Read the model definition and answer for the solid it produces. Units are mm, in the model's axes. Round coordinates to 2 decimals unless told otherwise and drop trailing zeros. Loops run counter-clockwise (first coordinate to the right, second up) from the corner with the lowest first, then second, coordinate; pieces in that order, holes last. Notation, with made-up numbers: (-37.75, 32) -> (-33.75, 32) arc R13 cw to (-33.75, 38) -> close; hole circle Ø9 at (40.25, -36.75). An arc over 180 degrees is marked (long way). Put each result on its own line as item: value.
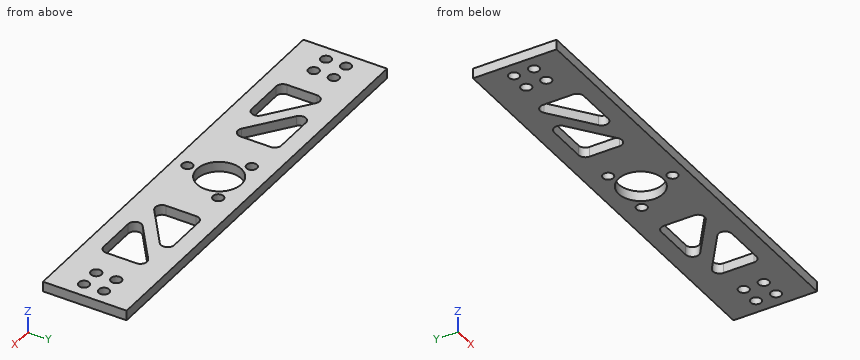
from build123d import *

# Parameters (mm, degrees)
SKETCH_1_W          = 127.5
SKETCH_1_H          = 25
EXTRUDE_1_DEPTH     = 3
SKETCH_2_R          = 1.575
SKETCH_2_R_2        = 6.65
CUT_EXTRUDE_1_DEPTH = 130.96249459
FILLET_1_R          = 2


with BuildPart() as part:
    # 草图1 → 凸台-拉伸1 (new body)
    with BuildSketch(Plane.XY):
        with Locations((63.75, -12.5)):
            Rectangle(SKETCH_1_W, SKETCH_1_H)
    extrude(amount=EXTRUDE_1_DEPTH)

    # 草图2 → 切除-拉伸1 (cut, through all)
    with BuildSketch(Plane.XY.offset(3)):
        with Locations((4.5, -9.5)):
            Circle(SKETCH_2_R)
        with Locations(Location((10.5, -9.5, 0), (0, 0, 180))):
            Circle(SKETCH_2_R)
        with Locations((10.5, -15.5)):
            Circle(SKETCH_2_R)
        with Locations(Location((4.5, -15.5, 0), (0, 0, 180))):
            Circle(SKETCH_2_R)
        with Locations((123, -15.5)):
            Circle(SKETCH_2_R)
        with Locations(Location((117, -15.5, 0), (0, 0, 180))):
            Circle(SKETCH_2_R)
        with Locations((117, -9.5)):
            Circle(SKETCH_2_R)
        with Locations(Location((123, -9.5, 0), (0, 0, 180))):
            Circle(SKETCH_2_R)
        with Locations((63.75, -11.25)):
            Circle(SKETCH_2_R_2)
        with Locations((55.522758664, -6.5)):
            Circle(SKETCH_2_R)
        with Locations((71.977241336, -6.5)):
            Circle(SKETCH_2_R)
        with Locations((63.75, -20.75)):
            Circle(SKETCH_2_R)
        Polygon((108, -5), (108, -20), (88, -20), align=None)
        Polygon((81.977241336, -5), (81.977241336, -20), (101.977241336, -5), align=None)
        Polygon((25.522758664, -5), (45.522758664, -5), (45.522758664, -20), align=None)
        Polygon((39.5, -20), (19.5, -5), (19.5, -20), align=None)
    extrude(amount=-CUT_EXTRUDE_1_DEPTH, mode=Mode.SUBTRACT)

    # 圆角1
    fillet_1_edges = [part.edges().sort_by_distance(p)[0] for p in [
        (45.522758664, -20, 1.5),
        (25.522758664, -5, 1.5),
        (45.522758664, -5, 1.5),
        (39.5, -20, 1.5),
        (19.5, -20, 1.5),
        (19.5, -5, 1.5),
        (81.977241336, -5, 1.5),
        (101.977241336, -5, 1.5),
        (81.977241336, -20, 1.5),
        (88, -20, 1.5),
        (108, -5, 1.5),
        (108, -20, 1.5),
    ]]
    fillet(fillet_1_edges, radius=FILLET_1_R)


solid = part.part
Item 1: The part is cut by section A-A (x = 88). Determine the outline of the cut face in (y, z), then the cut area to 3 significant figures.
Derived:
outline: (-25, 0) -> (-15.48, 0) -> (-15.48, 3) -> (-25, 3) -> close; (-5, 0) -> (0, 0) -> (0, 3) -> (-5, 3) -> close
area: 43.6 mm^2
Item 2: Find the intervals of material crossed by line 1 along Y through (x, z) = (10.5, 1.9) (3 decimals); line 2 along Y through (x, z) = (97, 2.8); line 3 along Y through (x, z) = (21.5, 2.3), in increasing order.
Derived:
line 1: y = -25 to -17.075, -13.925 to -11.075, -7.925 to 0
line 2: y = -25 to -20, -13.25 to -8.73, -5.28 to 0
line 3: y = -25 to -20, -7 to 0
Item 3: The part is cut by section C-C (z = 1.75). State how many separate pieces and enclosed holes the cut face has, then the cut area to 3 significant figures.
Derived:
separate pieces: 1
enclosed holes: 16
area: 2,410 mm^2
Item 4: The part is cut by section D-D (x = 27). Determine the outline of the cut face in (y, z) (3 decimals).
Derived:
outline: (-25, 0) -> (-20, 0) -> (-20, 3) -> (-25, 3) -> close; (-10.625, 0) -> (0, 0) -> (0, 3) -> (-10.625, 3) -> close
Item 5: The part is cut by section B-B (x = 4.5). Determine the outline of the cut face in (y, z) (3 decimals).
Derived:
outline: (-25, 0) -> (-17.075, 0) -> (-17.075, 3) -> (-25, 3) -> close; (-13.925, 0) -> (-11.075, 0) -> (-11.075, 3) -> (-13.925, 3) -> close; (-7.925, 0) -> (0, 0) -> (0, 3) -> (-7.925, 3) -> close
Item 6: Flat-ended cylindrical pins translate along their axes: pin 1 Ø4 at (x, y) = (10.5, -15.5) entering from +Z; pin 2 Ø3 at (x, y) = (63.75, -20.75) entering from -Z. Find the tip coordinate at first contact, or state that the pin passes through.
Derived:
pin 1: stops at z = 3
pin 2: passes through
